```python
from build123d import *

# Parameters (mm, degrees)
CUT_EXTRUDE3_START = -211
SKETCH21_R         = 5
CUT_EXTRUDE3_DEPTH = 231.0500001


with BuildPart() as part:
    # Sweep-Thin3: sweep along a curve in space
    with BuildLine() as sweep_thin3_path:
        Line((0, 0, 0), (-50, 0, 0))
        Line((0, 0, 0), (245.484298454, 0, 0))
        ThreePointArc((254.442631788, 0, 0.809063194), (249.981695461, 0, 0.202676576), (245.484298454, 0, 0))
        Line((254.442631788, 0, 0.809063194), (810.776679593, 0, 102.125))
        ThreePointArc((840.291241677, -30, 107.5), (831.646626586, -8.786796564, 105.925698949), (810.776679593, 0, 102.125))
        Line((840.291241677, -30, 107.5), (840.291241677, -210, 107.5))
    # Sketch2 → Sweep-Thin3 (sweep)
    with BuildSketch(Plane(origin=(0, 0, 0), x_dir=(0, 0, -1), z_dir=(1, 0, 0))):
        with BuildLine():
            Line((14.05, 19.05), (-14.05, 19.05))
            ThreePointArc((-14.05, 19.05), (-17.585533906, 17.585533906), (-19.05, 14.05))
            Line((-19.05, 14.05), (-19.05, -14.05))
            ThreePointArc((-19.05, -14.05), (-17.585533906, -17.585533906), (-14.05, -19.05))
            Line((-14.05, -19.05), (14.05, -19.05))
            ThreePointArc((14.05, -19.05), (17.585533906, -17.585533906), (19.05, -14.05))
            Line((19.05, -14.05), (19.05, 14.05))
            ThreePointArc((19.05, 14.05), (17.585533906, 17.585533906), (14.05, 19.05))
        make_face()
        with BuildLine():
            Line((14.05, 15.875), (-14.05, 15.875))
            ThreePointArc((-14.05, 15.875), (-15.340469876, 15.340469876), (-15.875, 14.05))
            Line((-15.875, 14.05), (-15.875, -14.05))
            ThreePointArc((-15.875, -14.05), (-15.340469876, -15.340469876), (-14.05, -15.875))
            Line((-14.05, -15.875), (14.05, -15.875))
            ThreePointArc((14.05, -15.875), (15.340469876, -15.340469876), (15.875, -14.05))
            Line((15.875, -14.05), (15.875, 14.05))
            ThreePointArc((15.875, 14.05), (15.340469876, 15.340469876), (14.05, 15.875))
        make_face(mode=Mode.SUBTRACT)
    sweep_thin3 = sweep(path=sweep_thin3_path.line)

    # Sketch21 → Cut-Extrude3 (cut)
    with BuildSketch(Plane(origin=(0, 0, 0), x_dir=(1, 0, 0), z_dir=(0, 1, 0)).offset(CUT_EXTRUDE3_START)):
        with Locations((50, 0)):
            Circle(SKETCH21_R)
    cut_extrude3 = extrude(amount=CUT_EXTRUDE3_DEPTH, mode=Mode.SUBTRACT)

    # Mirror1: Sweep-Thin3, Cut-Extrude3 across plane
    add(sweep_thin3.mirror(Plane(origin=(0, -210, 0), x_dir=(0, 0, 1), z_dir=(0, -1, 0))))
    add(cut_extrude3.mirror(Plane(origin=(0, -210, 0), x_dir=(0, 0, 1), z_dir=(0, -1, 0))), mode=Mode.SUBTRACT)


solid = part.part
```
Work out the finished part from the listing and answer in its coordinate system (mm). A direction names the side the tool comes from. Coordinates: 2 decimals unless noted, no trailing zeros. Loops run counter-clockwise (first coordinate to the right, second up) from the corner with the lowest first, then second, coordinate; pieces in that order, holes last. Notation, with made-up numbers: (7.5, 10.5) -> (56.5, 10.5) arc R20 ccw to (56.5, 20.5) -> close; hole circle Ø1 at (84.25, 82). An arc over 180 degrees is marked (long way). Answer as CSV lines item,"result".
Q1. For a pull along Z with two mould halves and no side action, classify faces 4 (the face through (96, -420, -19.05)), 5 (the face through (96, 0, 19.05)), 6 (the face through (353, -435.875, 6)) as +Z half, -Z half, draft (parallel to the pull), parting line (faces both ways), or undercut.
Findings:
face 4,"-Z half"
face 5,"+Z half"
face 6,"undercut"
Q2. A tool of negligible diameter and unlimited length cuts with its end or side. For faces 1 (the face through (818.51, -397.66, 103.33)), 2 (the face through (96, -420, 15.875)), 3 (the face through (843.075, -422.08, 107.807)), from which of +Z, -Z, +X, -X, +Y, -Y can it reach the whole face along a straight path? Write none if from no direction.
Findings:
face 1,"-Z, -X"
face 2,"-X"
face 3,"none"
Q3. The part is cut by section B-B on y = -132.5. Write down the section's boundary in (x, z) (3 decimals).
Findings:
outline,"(819.032, 117.91) -> (824.067, 90.264) arc R5 ccw to (829.882, 86.241) -> (857.527, 91.276) arc R5 ccw to (861.55, 97.09) -> (856.516, 124.736) arc R5 ccw to (850.701, 128.759) -> (823.055, 123.724) arc R5 ccw to start; hole (822.156, 118.478) -> (827.19, 90.833) arc R1.825 ccw to (829.313, 89.365) -> (856.958, 94.399) arc R1.825 ccw to (858.427, 96.522) -> (853.392, 124.167) arc R1.825 ccw to (851.27, 125.635) -> (823.624, 120.601) arc R1.825 ccw to start"
Q4. Each of these flat-tipped pins is pushed along its axis until it touches: pin 1 (8.5 mm diameter, centred on x = 170, y = -1, fed in from +Z); pin 2 (11.5 mm diameter, centred on x = 50, z = 0, fed in from +Y). Where does it stop, or does it pass through?
Findings:
pin 1,"stops at z = 19.05"
pin 2,"stops at y = 19.05"
Q5. Find the intervals of material crossed by probe 1 along Y at (x, z) = (307, 23) (3 decimals); probe 2 along Z at (x, y) = (40.5, -414) (3 decimals), in increasing order.
Findings:
probe 1,"y = -439.05 to -435.875, -404.125 to -400.95, -19.05 to -15.875, 15.875 to 19.05"
probe 2,"z = -19.05 to -15.875, 15.875 to 19.05"
Q6. The part is cut by section A-A on x = 197.5. State how many separate pieces and enclosed holes the cut face has, and give its area (3 significant figures).
Findings:
separate pieces,"2"
enclosed holes,"2"
area,"850 mm²"
